```python
from build123d import *

# Parameters (mm, degrees)
BOSS_EXTRUDE1_DEPTH = 20
FILLET1_R           = 10
CHAMFER1_SIZE       = 5
CHAMFER2_SIZE       = 5
BOSS_EXTRUDE2_DEPTH = 20
BOSS_EXTRUDE3_DEPTH = 20
BOSS_EXTRUDE4_DEPTH = 20
BOSS_EXTRUDE5_DEPTH = 20
SKETCH6_R           = 3.5
CUT_EXTRUDE1_DEPTH  = 20


with BuildPart() as part:
    # Sketch1 → Boss-Extrude1 (new body)
    with BuildSketch(Plane(origin=(0, 0, 0), x_dir=(1, 0, 0), z_dir=(0, 1, 0))):
        Polygon((-90, -12), (-90, -20), (90, -20), (90, 20), (-90, 20), (-90, 12), (80, 12), (80, -12), align=None)
    extrude(amount=BOSS_EXTRUDE1_DEPTH)

    # Fillet1
    fillet1_edges = [part.edges().sort_by_distance(p)[0] for p in [
        (80, 10, 12),
        (80, 10, -12),
    ]]
    fillet(fillet1_edges, radius=FILLET1_R)

    # Chamfer1
    chamfer1_edges = [part.edges().sort_by_distance(p)[0] for p in [
        (90, 10, 20),
        (90, 10, -20),
    ]]
    chamfer(chamfer1_edges, length=CHAMFER1_SIZE)

    # Chamfer2
    chamfer2_edges = [part.edges().sort_by_distance(p)[0] for p in [
        (-90, 10, 20),
        (-90, 10, -20),
    ]]
    chamfer(chamfer2_edges, length=CHAMFER2_SIZE)

    # Sketch2 → Boss-Extrude2 (add)
    with BuildSketch(Plane(origin=(0, 20, 0), x_dir=(1, 0, 0), z_dir=(0, 1, 0))):
        with BuildLine():
            Line((31.05572809, -12), (34, -12))
            ThreePointArc((34, -12), (40, -10), (46, -12))
            Line((46, -12), (48.94427191, -12))
            ThreePointArc((48.94427191, -12), (40, -8), (31.05572809, -12))
        make_face()
        with BuildLine():
            Line((31.05572809, 12), (34, 12))
            ThreePointArc((34, 12), (40, 10), (46, 12))
            Line((46, 12), (48.94427191, 12))
            ThreePointArc((48.94427191, 12), (40, 8), (31.05572809, 12))
        make_face()
    extrude(amount=-BOSS_EXTRUDE2_DEPTH)

    # Sketch3 → Boss-Extrude3 (add)
    with BuildSketch(Plane(origin=(0, 20, 0), x_dir=(1, 0, 0), z_dir=(0, 1, 0))):
        Polygon((85, 20), (83.468895387, 21.5), (82.097625423, 20.100294822), (80.668895387, 21.5), (79.297625423, 20.100294822), (77.868895387, 21.5), (76.497625423, 20.100294822), (75.068895387, 21.5), (73.697625423, 20.100294822), (72.268895387, 21.5), (70.897625423, 20.100294822), (69.468895387, 21.5), (68.097625423, 20.100294822), (66.668895387, 21.5), (65.297625423, 20.100294822), (63.868895387, 21.5), (62.497625423, 20.100294822), (61.068895387, 21.5), (59.697625423, 20.100294822), (58.268895387, 21.5), (56.897625423, 20.100294822), (55.468895387, 21.5), (54.097625423, 20.100294822), (52.668895387, 21.5), (51.297625423, 20.100294822), (49.868895387, 21.5), (48.497625423, 20.100294822), (47.068895387, 21.5), (45.697625423, 20.100294822), (44.268895387, 21.5), (42.799368105, 20), align=None)
    extrude(amount=-BOSS_EXTRUDE3_DEPTH)

    # Sketch4 → Boss-Extrude4 (add)
    with BuildSketch(Plane(origin=(0, 20, 0), x_dir=(1, 0, 0), z_dir=(0, 1, 0))):
        Polygon((83.5, -21.5), (85, -20), (42.8, -20), (44.3, -21.5), (45.7, -20.1), (47.1, -21.5), (48.5, -20.1), (49.9, -21.5), (51.3, -20.1), (52.7, -21.5), (54.1, -20.1), (55.5, -21.5), (56.9, -20.1), (58.3, -21.5), (59.7, -20.1), (61.1, -21.5), (62.5, -20.1), (63.9, -21.5), (65.3, -20.1), (66.7, -21.5), (68.1, -20.1), (69.5, -21.5), (70.9, -20.1), (72.3, -21.5), (73.7, -20.1), (75.1, -21.5), (76.5, -20.1), (77.9, -21.5), (79.3, -20.1), (80.7, -21.5), (82.1, -20.1), align=None)
    extrude(amount=-BOSS_EXTRUDE4_DEPTH)

    # Sketch5 → Boss-Extrude5 (add)
    with BuildSketch(Plane(origin=(0, 20, 0), x_dir=(1, 0, 0), z_dir=(0, 1, 0))):
        Polygon((90, 15), (97, 8), (97, -8), (90, -15), align=None)
    extrude(amount=-BOSS_EXTRUDE5_DEPTH)

    # Sketch6 → Cut-Extrude1 (cut)
    with BuildSketch(Plane(origin=(0, 20, 0), x_dir=(1, 0, 0), z_dir=(0, 1, 0))):
        with Locations(Location((89, 0, 0), (0, 0, 270))):
            Circle(SKETCH6_R)
    extrude(amount=-CUT_EXTRUDE1_DEPTH, mode=Mode.SUBTRACT)


solid = part.part
```
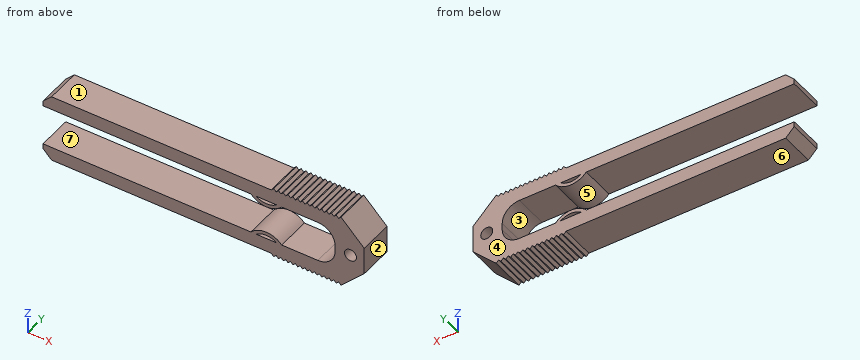
CAD build for the part. Positions are in the model's coordinates, mm. Face numbers are marked on the shaded views. A direction names the side the tool comes from. Round coordinates to 2 decimals unless told otherwise and drop trailing zeros. Loops run counter-clockwise (first coordinate to the right, second up) from the corner with the lowest first, then second, coordinate; pieces in that order, holes last. Notation, with made-up numbers: M -6,0.5 L 8,0.5 A36 cw 8,38.5 Z; hole C 85,31.5 d7. An arc over 180 degrees is marked long. Return JSON: item names as keys, results as strings. Group by question number.
(1) Saw through at D-D, the plane z = -18. List the corners of the cut face in (x, y), and give its area (3 significant figures).
(2) Saw through at B-B, the plane x = 89. List the corners of the cut face in (y, z).
(3) Drop flat-ended pins along their axis: P1, Ø5, axis at y = 10.5, z = -13, coming from the +X side; P2, Ø9.5, axis at x = 40, y = 14.5, coming from the +Z side; P3, Ø12, axis at x = 25, y = 13, coming from the -Z side. Give the stop position or say it passes through.
(4) Saw through at A-A, the plane z = 0. List the corners of the cut face in (x, y).
(5) Tool access for the marked faces 4, 5, 6 and 7: list every direction of +Z, -Z, +X, -X, +Y, -Y with a clear straight run to the whole face (end or side of a thin tool).
(6) Wall check: probe 1 along Z at (x, y) = (2.5, 3.25); probe 2 along Z at (x, y) = (42, 17); probe 3 along X at (y, z) = (6.25, 0). Give the ranges that are in metal, low to high. Write a range as [from, to].
(7) Saw through at C-C, the plane y = 17.75. Give the number of separate pieces and of enclosed holes in the cut face, and give its area (3 significant figures).
(8) Mould opens along Z. For the marked faces 1, 2 and 3 say: +Z half, -Z half, draft (parallel to the pull), parting line (faces both ways), or undercut.
Answer list:
{
 "1": {"outline": "M -87,0 L 87,0 L 87,20 L -87,20 Z", "area": "3,480 mm2"},
 "2": {"outline": "M 0,-16 L 20,-16 L 20,-3.5 L 0,-3.5 Z; M 0,3.5 L 20,3.5 L 20,16 L 0,16 Z"},
 "3": {"P1": "x = 94.5", "P2": "z = 21.5", "P3": "z = -20"},
 "4": {"outline": "M 80,0 L 85.5,0 L 85.5,20 L 80,20 Z; M 92.5,0 L 97,0 L 97,20 L 92.5,20 Z"},
 "5": {"face 4": "+Z, -Z, +X, -X, +Y", "face 5": "+Y, -Y", "face 6": "-Z, -X, +Y, -Y", "face 7": "-X, +Y, -Y"},
 "6": {"probe 1": "[-20, -12], [12, 20]", "probe 2": "[-20, -12], [-10.2, -8.17], [8.17, 10.2], [12, 20]", "probe 3": "[80, 85.5], [92.5, 97]"},
 "7": {"separate pieces": "1", "enclosed holes": "3", "area": "3,370 mm2"},
 "8": {"face 1": "+Z half", "face 2": "draft", "face 3": "undercut"}
}
